Geometry: final body of the model. Coordinates: model frame, mm. A direction names the side the tool comes from. Give positions to 0.01 mm unless a question says otherwise; leave off trailing zeros. Order: outer loops, then holes, each group sorted by start corner. A loop starts at its lowest first (then second) coordinate and runs counter-clockwise, first axis right, second up. Notation, with made-up numbers: (89, 88) -> (133, 88) arc R26 cw to (133, 112) -> close; hole circle Ø4 at (88, -23). An arc over 180 degrees is marked (long way). One line per question, with ' | ' between items.
from build123d import *

# Parameters (mm, degrees)
SKETCH1_W           = 10
SKETCH1_H           = 10
BOSS_EXTRUDE1_DEPTH = 50
SKETCH2_W           = 7
SKETCH2_H           = 44
CUT_EXTRUDE1_DEPTH  = 11
SKETCH3_R           = 2
CUT_EXTRUDE2_DEPTH  = 71


with BuildPart() as part:
    # Sketch1 → Boss-Extrude1 (new body)
    with BuildSketch(Plane.XY):
        Rectangle(SKETCH1_W, SKETCH1_H)
    extrude(amount=BOSS_EXTRUDE1_DEPTH)

    # Sketch2 → Cut-Extrude1 (cut)
    with BuildSketch(Plane(origin=(0, 5, 0), x_dir=(1, 0, 0), z_dir=(0, 1, 0))):
        with Locations((1.5, -25)):
            Rectangle(SKETCH2_W, SKETCH2_H)
    extrude(amount=-CUT_EXTRUDE1_DEPTH, mode=Mode.SUBTRACT)

    # Sketch3 → Cut-Extrude2 (cut)
    with BuildSketch(Plane.XY.offset(50)):
        with Locations((1.5, 0)):
            Circle(SKETCH3_R)
    extrude(amount=-CUT_EXTRUDE2_DEPTH, mode=Mode.SUBTRACT)


solid = part.part
1) Set-up query: faces 1 (the flat face through (-2, 0, 25)), 2 (the flat face through (5, 0, 48)). Return all of +Z, -Z, +X, -X, +Y, -Y with unobstructed straight access to the full face (end or side cutting, diameter ignored); none if empty.
Check result:
face 1: +X, +Y, -Y | face 2: +Z, -Z, +X, +Y, -Y
2) Section B-B on x = 1.5. Return loops of the section in (y, z), plus the area to 3 significant figures.
Check result:
outline: (-5, 0) -> (-2, 0) -> (-2, 3) -> (-5, 3) -> close; (-5, 47) -> (-2, 47) -> (-2, 50) -> (-5, 50) -> close; (2, 0) -> (5, 0) -> (5, 3) -> (2, 3) -> close; (2, 47) -> (5, 47) -> (5, 50) -> (2, 50) -> close | area: 36.0 mm^2
3) Pull-direction query (Z, two-part tool) for faces 3 (the flat face through (-1, 0, 0)), 4 (the flat face through (1.5, 2.3, 3)), 5 (the cylindrical face through (2.423, -1.774, 1.521)); classes: +Z half, -Z half, draft (parallel to the pull), parting line (faces both ways), or undercut.
Check result:
face 3: -Z half | face 4: undercut | face 5: draft
4) Section C-C on y = 3.5. Return loops of the section in (x, z).
Check result:
outline: (-5, 0) -> (5, 0) -> (5, 3) -> (-2, 3) -> (-2, 47) -> (5, 47) -> (5, 50) -> (-5, 50) -> close
5) Section A-A on y = 0. Return loops of the section in (x, z).
Check result:
outline: (-5, 0) -> (-0.5, 0) -> (-0.5, 3) -> (-2, 3) -> (-2, 47) -> (-0.5, 47) -> (-0.5, 50) -> (-5, 50) -> close; (3.5, 0) -> (5, 0) -> (5, 3) -> (3.5, 3) -> close; (3.5, 47) -> (5, 47) -> (5, 50) -> (3.5, 50) -> close
6) Material intervals for probe 1 along Z at (x, y) = (1.75, 4.75); probe 2 along Y at (x, z) = (1.5, 1.25); probe 3 along X at (y, z) = (-4, 6.5), sorted ascending. Write a range as from..to.
Check result:
probe 1: z = 0..3, 47..50 | probe 2: y = -5..-2, 2..5 | probe 3: x = -5..-2
7) Section D-D on z = 42.5. Return loops of the section in (x, y).
Check result:
outline: (-5, -5) -> (-2, -5) -> (-2, 5) -> (-5, 5) -> close
8) Contact query for flat-ended pins moving along their axis: pin 1 Ø5 at (x, y) = (0.5, 0.5) entering from +Z; pin 2 Ø3 at (y, z) = (-2, 30.5) entering from +X. Output: stop coordinate, or through.
Check result:
pin 1: stops at z = 50 | pin 2: stops at x = -2
